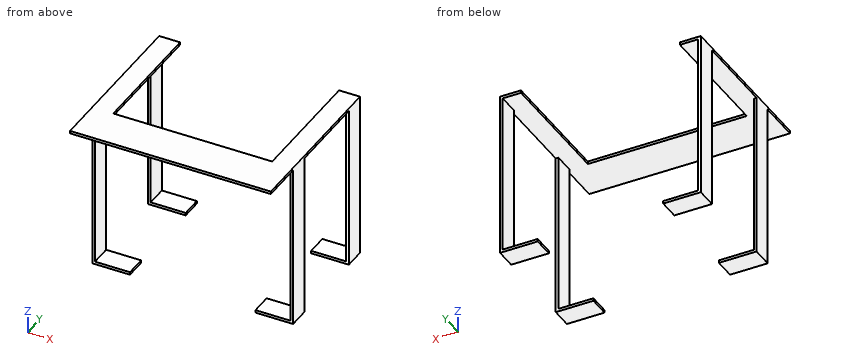
```python
from build123d import *

# Parameters (mm, degrees)
F0_W     = 60.96
F0_H     = 50.8
F1_DEPTH = 0.8128
F2_W     = 48.26
F2_H     = 38.1
F3_DEPTH = 25.4
F4_W     = 0.8128
F4_H     = 6.35
F5_DEPTH = 50.8
F6_W     = 6.35
F6_H     = 0.8128
F7_DEPTH = 11.43
F8_W     = 6.35
F8_H     = 0.8128
F9_DEPTH = 11.43


with BuildPart() as f1:
    # F0 (on Top) → F1 (new body)
    with BuildSketch(Plane.XY):
        with Locations((30.48, 25.4)):
            Rectangle(F0_W, F0_H)
    extrude(amount=F1_DEPTH)

    # F2 (on face) → F3 (cut)
    with BuildSketch(Plane.XY.offset(0.8128)):
        with Locations((30.48, 31.75)):
            Rectangle(F2_W, F2_H)
    extrude(amount=-F3_DEPTH, mode=Mode.SUBTRACT)

    # F4 (on face) → F5 (join)
    with BuildSketch(Plane.XY.offset(0.8128)):
        with Locations((0.4064, 47.625)):
            Rectangle(F4_W, F4_H)
        with Locations((60.5536, 47.625)):
            Rectangle(F4_W, F4_H)
        with Locations((0.4064, 15.875)):
            Rectangle(F4_W, F4_H)
        with Locations((60.5536, 15.875)):
            Rectangle(F4_W, F4_H)
    extrude(amount=-F5_DEPTH)

    # F6 (on face) → F7 (join)
    with BuildSketch(Plane.YZ.offset(60.96)):
        with Locations((15.875, -49.5808)):
            Rectangle(F6_W, F6_H)
        with Locations((47.625, -49.5808)):
            Rectangle(F6_W, F6_H)
    extrude(amount=-F7_DEPTH)

    # F8 (on face) → F9 (join)
    with BuildSketch(Plane(origin=(0, 0, 0), x_dir=(0, -1, 0), z_dir=(-1, 0, 0))):
        with Locations((-47.625, -49.5808)):
            Rectangle(F8_W, F8_H)
        with Locations((-15.875, -49.5808)):
            Rectangle(F8_W, F8_H)
    extrude(amount=-F9_DEPTH)


solid = f1.part
```
The model under review builds one solid part; all positions refer to its coordinate system, in mm. Round coordinates to 2 decimals unless told otherwise and drop trailing zeros. Order: outer loops, then holes, each group sorted by start corner. A loop starts at its lowest first (then second) coordinate and runs counter-clockwise, first axis right, second up.
Item 1: For pin 1 (9 mm diameter, centred on x = 57.5, z = -22, fed in from -Y); pin 2 (1 mm diameter, centred on x = 54.5, y = 41.5, fed in from -Z), all flat-tipped, find the tip position at first contact; note any pin that passes through.
Working result:
pin 1: stops at y = 12.7
pin 2: stops at z = 0
Item 2: Add section D-D, the plane y = 7.5. State the section outline as (x, z) points.
Working result:
outline: (0, 0) - (60.96, 0) - (60.96, 0.81) - (0, 0.81) - close
Item 3: To check wall thickness, follow probe 1 along X at (y, z) = (16, -13); probe 2 along Z at (x, y) = (22, 3.5). State the ranges of each line that lie inside material, in increasing order.
Working result:
probe 1: x = 0 to 0.81, 60.15 to 60.96
probe 2: z = 0 to 0.81
Item 4: Add section A-A, the plane x = 57.5. State the section outline as (y, z) points, and give its area (3 significant figures).
Working result:
outline: (0, 0) - (50.8, 0) - (50.8, 0.81) - (0, 0.81) - close; (12.7, -49.99) - (19.05, -49.99) - (19.05, -49.17) - (12.7, -49.17) - close; (44.45, -49.99) - (50.8, -49.99) - (50.8, -49.17) - (44.45, -49.17) - close
area: 51.6 mm2
Item 5: Add section B-B, the plane y = 36. State the section outline as (x, z) points, and give its area (3 significant figures).
Working result:
outline: (0, 0) - (6.35, 0) - (6.35, 0.81) - (0, 0.81) - close; (54.61, 0) - (60.96, 0) - (60.96, 0.81) - (54.61, 0.81) - close
area: 10.3 mm2
Item 6: Add section C-C, the plane z = -23. State the section outline as (x, y) points.
Working result:
outline: (0, 12.7) - (0.81, 12.7) - (0.81, 19.05) - (0, 19.05) - close; (0, 44.45) - (0.81, 44.45) - (0.81, 50.8) - (0, 50.8) - close; (60.15, 12.7) - (60.96, 12.7) - (60.96, 19.05) - (60.15, 19.05) - close; (60.15, 44.45) - (60.96, 44.45) - (60.96, 50.8) - (60.15, 50.8) - close
